Verification items for the finished model (mm, model axes). Face numbers are marked on the shaded views. Give positions to 0.01 mm unless a question says otherwise; leave off trailing zeros. Write each loop counter-clockwise with the first axis right and the second up, starting at its lowest first coordinate (ties: lowest second). Pieces come first, ordered by that corner, then holes. Notation, with made-up numbers: (47.25, 15.5) - (56.25, 15.5) arc R13 ccw to (56.25, 30.5) - close; hole circle Ø10 at (53, 64). An arc over 180 degrees is marked (long way). Answer as a JSON object with one key per item and string values. Group by question number.
Item 1: Go/stop test with flat-tipped pins: pin 1 (9.5 mm diameter, centred on y = -517, z = 10.5, fed in from -X); pin 2 (20.5 mm diameter, centred on y = -315.5, z = 39.5, fed in from -X); pin 3 (5 mm diameter, centred on y = 3.5, z = 12.5, fed in from +X). Record where each tip stops, or that it passes through.
Item 2: Sectioned sample at D-D, the plane x = -1416. Record the boundary of the cut face in (y, z).
Item 3: Sectioned sample at A-A, the plane y = 209. Count the separate pieces of the cut face and the enclosed holes in it, and give its area (3 significant figures).
Item 4: Sectioned sample at B-B, the plane z = 40.5. Record the boundary of the cut face in (x, y), and give its area (3 significant figures).
Item 5: Sectioned sample at C-C, the plane x = -331.5. Record the boundary of the cut face in (y, z).
Item 6: Draft check along Y on the marked faces 1 and 2. Enter one of: +Y half, -Y half, draft (parallel to the pull), parting line (faces both ways), or undercut.
Item 7: Scan lines: line 1 along Y through (x, z) = (-196.5, 19); line 2 along Y through (x, z) = (-1300, 11); line 3 along Y through (x, z) = (-2115.5, 37). Record each from-to range of solid material in increasing order. Write a range as [from, to].
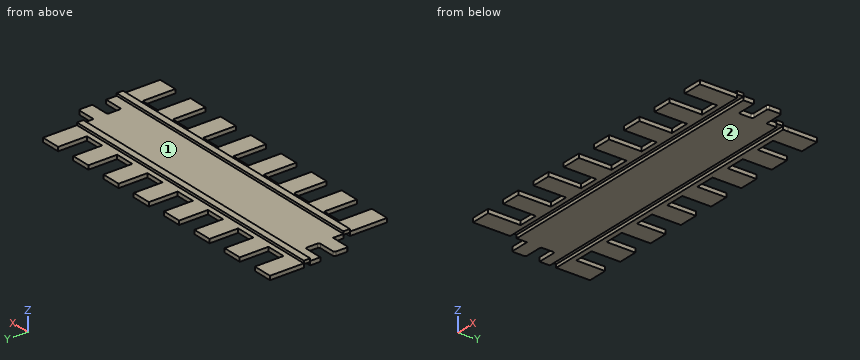
```python
from build123d import *

# Parameters (mm, degrees)
F2_DEPTH = 31.75
F1_W     = 2314.8620128632
F1_H     = 50.8
F1_W_2   = 2314.7030770779
F3_DEPTH = 50.8
F5_DEPTH = 25.4


with BuildPart() as f2:
    # F0 (on Top) → F2 (new body)
    with BuildSketch(Plane.XY):
        with BuildLine():
            Line((141.605, 0), (0, 0))
            Line((0, 0), (-0.0174862289, 172.1356511116))
            Line((-0.0174862289, 172.1356511116), (-0.0174862289, 400.9649455547))
            Line((-0.0174862289, 400.9649455547), (-154.3224862289, 400.9649455547))
            Line((-154.3224862289, 400.9649455547), (-154.3224862289, 172.1356511116))
            Line((-154.3224862289, 172.1356511116), (-308.6274862289, 172.1356511116))
            Line((-308.6274862289, 172.1356511116), (-308.6274862289, 400.9649455547))
            Line((-308.6274862289, 400.9649455547), (-462.9324862289, 400.9649455547))
            Line((-462.9324862289, 400.9649455547), (-462.9324862289, 172.1356511116))
            Line((-462.9324862289, 172.1356511116), (-617.2374862289, 172.1356511116))
            Line((-617.2374862289, 172.1356511116), (-617.2374862289, 400.9649455547))
            Line((-617.2374862289, 400.9649455547), (-771.5424862289, 400.9649455547))
            Line((-771.5424862289, 400.9649455547), (-771.5424862289, 172.1356511116))
            Line((-771.5424862289, 172.1356511116), (-925.8474862289, 172.1356511116))
            Line((-925.8474862289, 172.1356511116), (-925.8474862289, 400.9649455547))
            Line((-925.8474862289, 400.9649455547), (-1080.1524862289, 400.9649455547))
            Line((-1080.1524862289, 400.9649455547), (-1080.1524862289, 172.1356511116))
            Line((-1080.1524862289, 172.1356511116), (-1234.4574862289, 172.1356511116))
            Line((-1234.4574862289, 172.1356511116), (-1234.4574862289, 400.9649455547))
            Line((-1234.4574862289, 400.9649455547), (-1388.7624862289, 400.9649455547))
            Line((-1388.7624862289, 400.9649455547), (-1388.7624862289, 172.1356511116))
            Line((-1388.7624862289, 172.1356511116), (-1543.0674862289, 172.1356511116))
            Line((-1543.0674862289, 172.1356511116), (-1543.0674862289, 399.8836874962))
            Line((-1543.0674862289, 399.8836874962), (-1697.3724862289, 399.8836874962))
            Line((-1697.3724862289, 399.8836874962), (-1697.3724862289, 172.1356511116))
            Line((-1697.3724862289, 172.1356511116), (-1851.6774862289, 172.1356511116))
            Line((-1851.6774862289, 172.1356511116), (-1851.6774862289, 399.8836874962))
            Line((-1851.6774862289, 399.8836874962), (-2005.9824862289, 399.8836874962))
            Line((-2005.9824862289, 399.8836874962), (-2005.9824862289, 172.1356511116))
            Line((-2005.9824862289, 172.1356511116), (-2160.2874862289, 172.1356511116))
            Line((-2160.2874862289, 172.1356511116), (-2160.2874862289, 399.8836874962))
            Line((-2160.2874862289, 399.8836874962), (-2314.5924862289, 399.8836874962))
            Line((-2314.5924862289, 399.8836874962), (-2314.5924862289, 0))
            Line((-2314.5924862289, 0), (-2172.9874862289, 0))
            ThreePointArc((-2172.9874862289, 0), (-2164.0072301079, -3.7197438789), (-2160.2874862289, -12.7))
            Line((-2160.2874862289, -12.7), (-2160.2874862289, -97.307886156))
            ThreePointArc((-2160.2874862289, -97.307886156), (-2164.0072301079, -106.2881422771), (-2172.9874862289, -110.007886156))
            Line((-2172.9874862289, -110.007886156), (-2301.8924862289, -110.007886156))
            ThreePointArc((-2301.8924862289, -110.007886156), (-2310.87274235, -113.7276300349), (-2314.5924862289, -122.707886156))
            Line((-2314.5924862289, -122.707886156), (-2314.5924862289, -207.315286156))
            ThreePointArc((-2314.5924862289, -207.315286156), (-2310.87274235, -216.2955422771), (-2301.8924862289, -220.015286156))
            Line((-2301.8924862289, -220.015286156), (-2160.2874862289, -220.015286156))
            Line((-2160.2874862289, -220.015286156), (-2160.2874862289, -647.8700637817))
            Line((-2160.2874862289, -647.8700637817), (-2005.9736835098, -647.8700637817))
            Line((-2005.9736835098, -647.8700637817), (-2005.9736835098, -389.8174464703))
            Line((-2005.9736835098, -389.8174464703), (-1851.6686835098, -389.8174464703))
            Line((-1851.6686835098, -389.8174464703), (-1851.6686835098, -647.8700637817))
            Line((-1851.6686835098, -647.8700637817), (-1697.355, -647.8700637817))
            Line((-1697.355, -647.8700637817), (-1697.355, -389.8174464703))
            Line((-1697.355, -389.8174464703), (-1543.05, -389.8174464703))
            Line((-1543.05, -389.8174464703), (-1543.05, -647.8700637817))
            Line((-1543.05, -647.8700637817), (-1388.745, -647.8700637817))
            Line((-1388.745, -647.8700637817), (-1388.745, -389.8174464703))
            Line((-1388.745, -389.8174464703), (-1234.44, -389.8174464703))
            Line((-1234.44, -389.8174464703), (-1234.44, -647.8700637817))
            Line((-1234.44, -647.8700637817), (-1080.135, -647.8700637817))
            Line((-1080.135, -647.8700637817), (-1080.135, -389.8174464703))
            Line((-1080.135, -389.8174464703), (-925.83, -389.8174464703))
            Line((-925.83, -389.8174464703), (-925.83, -647.8700637817))
            Line((-925.83, -647.8700637817), (-771.525, -647.8700637817))
            Line((-771.525, -647.8700637817), (-771.525, -389.8174464703))
            Line((-771.525, -389.8174464703), (-617.22, -389.8174464703))
            Line((-617.22, -389.8174464703), (-617.22, -647.8700637817))
            Line((-617.22, -647.8700637817), (-462.915, -647.8700637817))
            Line((-462.915, -647.8700637817), (-462.915, -389.8174464703))
            Line((-462.915, -389.8174464703), (-308.61, -389.8174464703))
            Line((-308.61, -389.8174464703), (-308.61, -647.8700637817))
            Line((-308.61, -647.8700637817), (-154.305, -647.8700637817))
            Line((-154.305, -647.8700637817), (-154.305, -389.8174464703))
            Line((-154.305, -389.8174464703), (0, -389.8174464703))
            Line((0, -389.8174464703), (0, -647.8700637817))
            Line((0, -647.8700637817), (154.305, -647.8700637817))
            Line((154.305, -647.8700637817), (154.305, -220.015286156))
            Line((154.305, -220.015286156), (12.7, -220.015286156))
            ThreePointArc((12.7, -220.015286156), (3.7197438789, -216.2955422771), (0, -207.315286156))
            Line((0, -207.315286156), (0, -122.707886156))
            ThreePointArc((0, -122.707886156), (3.7197438789, -113.7276300349), (12.7, -110.007886156))
            Line((12.7, -110.007886156), (141.605, -110.007886156))
            ThreePointArc((141.605, -110.007886156), (150.5852561211, -106.2881422771), (154.305, -97.307886156))
            Line((154.305, -97.307886156), (154.305, -12.7))
            ThreePointArc((154.305, -12.7), (150.5852561211, -3.7197438789), (141.605, 0))
        make_face()
    extrude(amount=F2_DEPTH)

    # F1 (on face) → F3 (join)
    with BuildSketch(Plane.XY):
        with Locations((-1157.4310064316, 106.5107680202)):
            Rectangle(F1_W, F1_H)
        with Locations((-1003.2348185778, -327.8856937885)):
            Rectangle(F1_W_2, F1_H)
    extrude(amount=F3_DEPTH)

    # F4 (on face) → F5 (cut)
    with BuildSketch(Plane(origin=(0, 0, 0), x_dir=(1, 0, 0), z_dir=(0, 0, -1))):
        Polygon((-2314.8620128632, -131.9107680202), (-2314.5924862289, -131.9107680202), (-0.0134000242, -131.9107680202), (0, -131.9107680202), (0, -81.1107680202), (-0.0082395567, -81.1107680202), (-2314.5924862289, -81.1107680202), (-2314.8620128632, -81.1107680202), align=None)
        Polygon((-2160.5863571167, 302.4856937885), (-2160.2874862289, 302.4856937885), (154.305, 302.4856937885), (154.305, 353.2856937885), (-2160.2874862289, 353.2856937885), (-2160.5863571167, 353.2856937885), align=None)
    extrude(amount=-F5_DEPTH, mode=Mode.SUBTRACT)


solid = f2.part
```
Geometry check:
{
 "1": {"pin 1": "x = -2160.29", "pin 2": "x = -2160.59", "pin 3": "x = 0"},
 "2": {"outline": "(-647.87, 0) - (-353.29, 0) - (-353.29, 25.4) - (-302.49, 25.4) - (-302.49, 0) - (81.11, 0) - (81.11, 25.4) - (131.91, 25.4) - (131.91, 0) - (172.14, 0) - (172.14, 31.75) - (131.91, 31.75) - (131.91, 50.8) - (81.11, 50.8) - (81.11, 31.75) - (-302.49, 31.75) - (-302.49, 50.8) - (-353.29, 50.8) - (-353.29, 31.75) - (-647.87, 31.75) - close"},
 "3": {"separate pieces": "8", "enclosed holes": "0", "area": "39,200 mm^2"},
 "4": {"outline": "(-2314.86, 81.11) - (0, 81.11) - (0, 131.91) - (-2314.86, 131.91) - close; (-2160.59, -353.29) - (154.12, -353.29) - (154.12, -302.49) - (-2160.59, -302.49) - close", "area": "235,000 mm^2"},
 "5": {"outline": "(-389.82, 0) - (-353.29, 0) - (-353.29, 25.4) - (-302.49, 25.4) - (-302.49, 0) - (81.11, 0) - (81.11, 25.4) - (131.91, 25.4) - (131.91, 0) - (400.96, 0) - (400.96, 31.75) - (131.91, 31.75) - (131.91, 50.8) - (81.11, 50.8) - (81.11, 31.75) - (-302.49, 31.75) - (-302.49, 50.8) - (-353.29, 50.8) - (-353.29, 31.75) - (-389.82, 31.75) - close"},
 "6": {"face 1": "undercut", "face 2": "draft"},
 "7": {"line 1": "[-647.87, -353.29], [-302.49, 81.11], [131.91, 172.14]", "line 2": "[-389.82, -353.29], [-302.49, 81.11], [131.91, 400.96]", "line 3": "[-353.29, -302.49], [81.11, 131.91]"}
}
